```python
from build123d import *

# Parameters (mm, degrees)
SKETCH1_R           = 17.5
BOSS_EXTRUDE1_DEPTH = 10
CUT_EXTRUDE2_DEPTH  = 3
SKETCH4_R           = 17.5
CUT_EXTRUDE3_DEPTH  = 5
SKETCH5_R           = 1.6
CUT_EXTRUDE4_DEPTH  = 5


with BuildPart() as part:
    # Sketch1 → Boss-Extrude1 (new body)
    with BuildSketch(Plane(origin=(0, 0, 0), x_dir=(1, 0, 0), z_dir=(0, 1, 0))):
        with Locations(Location((0, 0, 0), (0, 0, 270))):
            Circle(SKETCH1_R)
    extrude(amount=BOSS_EXTRUDE1_DEPTH)

    # Sketch3 → Cut-Extrude2 (cut)
    with BuildSketch(Plane(origin=(-674.936170281, 10, -1288.963286539), x_dir=(1, 0, 0), z_dir=(0, 1, 0))):
        with BuildLine():
            Line((670.88481746, -1281.946137613), (662.239438243, -1279.26312032))
            add(Edge.make_bspline(
                [(662.239438243, -1279.26312032), (660.816630975, -1279.364358211), (659.786645841, -1280.216704525), (659.563484847, -1281.534870974), (660.187213896, -1282.817677158)],
                knots=[0.002399099, 0.002399099, 0.002399099, 0.375599775, 0.624400225, 0.997600901, 0.997600901, 0.997600901], degree=2))
            Line((660.187213896, -1282.817677158), (666.833464638, -1288.963286539))
            Line((666.833464638, -1288.963286539), (660.187213896, -1295.108895919))
            add(Edge.make_bspline(
                [(660.187213896, -1295.108895919), (659.563484847, -1296.391702103), (659.786645841, -1297.709868552), (660.816630975, -1298.562214867), (662.239438243, -1298.663452757)],
                knots=[0.002399099, 0.002399099, 0.002399099, 0.375599775, 0.624400225, 0.997600901, 0.997600901, 0.997600901], degree=2))
            Line((662.239438243, -1298.663452757), (670.88481746, -1295.980435464))
            Line((670.88481746, -1295.980435464), (672.883945934, -1304.809062138))
            add(Edge.make_bspline(
                [(672.883945934, -1304.809062138), (673.683024153, -1305.990630431), (674.936170281, -1306.456450565), (676.189316409, -1305.990630431), (676.988394628, -1304.809062138)],
                knots=[0.002399099, 0.002399099, 0.002399099, 0.375599775, 0.624400225, 0.997600901, 0.997600901, 0.997600901], degree=2))
            Line((676.988394628, -1304.809062138), (678.987523102, -1295.980435464))
            Line((678.987523102, -1295.980435464), (687.632902319, -1298.663452757))
            add(Edge.make_bspline(
                [(687.632902319, -1298.663452757), (689.055709587, -1298.562214867), (690.085694721, -1297.709868552), (690.308855715, -1296.391702103), (689.685126666, -1295.108895919)],
                knots=[0.002399099, 0.002399099, 0.002399099, 0.375599775, 0.624400225, 0.997600901, 0.997600901, 0.997600901], degree=2))
            Line((689.685126666, -1295.108895919), (683.038875923, -1288.963286539))
            Line((683.038875923, -1288.963286539), (689.685126666, -1282.817677158))
            add(Edge.make_bspline(
                [(689.685126666, -1282.817677158), (690.308855715, -1281.534870974), (690.08569472, -1280.216704525), (689.055709587, -1279.364358211), (687.632902319, -1279.26312032)],
                knots=[0.002399099, 0.002399099, 0.002399099, 0.375599775, 0.624400225, 0.997600901, 0.997600901, 0.997600901], degree=2))
            Line((687.632902319, -1279.26312032), (678.987523102, -1281.946137613))
            Line((678.987523102, -1281.946137613), (676.986708426, -1273.110064271))
            add(Edge.make_bspline(
                [(676.986708426, -1273.110064271), (676.173308063, -1271.410983092), (674.936170281, -1270.754606381), (673.699032499, -1271.410983092), (672.885632136, -1273.110064271)],
                knots=[0.001074269, 0.001074269, 0.001074269, 0.375268567, 0.624731433, 0.998925731, 0.998925731, 0.998925731], degree=2))
            Line((672.885632136, -1273.110064271), (670.88481746, -1281.946137613))
        make_face()
    extrude(amount=-CUT_EXTRUDE2_DEPTH, mode=Mode.SUBTRACT)

    # Sketch4 → Cut-Extrude3 (cut)
    with BuildSketch(Plane.XZ):
        with Locations(Location((0, 0, 0), (0, 0, 270))):
            Circle(SKETCH4_R)
    extrude(amount=-CUT_EXTRUDE3_DEPTH, mode=Mode.SUBTRACT)

    # Sketch5 → Cut-Extrude4 (cut)
    with BuildSketch(Plane(origin=(0, 7, 0), x_dir=(1, 0, 0), z_dir=(0, 1, 0))):
        with Locations(Location((0, 0, 0), (0, 0, 270))):
            Circle(SKETCH5_R)
    extrude(amount=-CUT_EXTRUDE4_DEPTH, mode=Mode.SUBTRACT)


solid = part.part
```
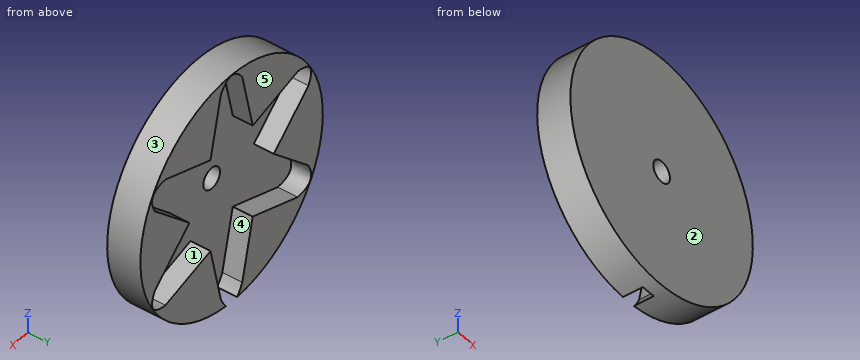
Input: part model. Units: mm. Frame: model coordinates. Face numbers are marked on the shaded views. A direction names the side the tool comes from. Coordinates: 2 decimals unless noted, no trailing zeros. Write each loop counter-clockwise with the first axis right and the second up, starting at its lowest first coordinate (ties: lowest second). Pieces come first, ordered by that corner, then holes.
1) Section D-D on z = 15. Output: boundary loops of the cut face in (x, y), and give its area (3 significant figures).
2) Section A-A on y = 5.9. Output: boundary loops of the cut face in (x, z).
3) Set-up query: the marked faces 1 and 2. Return all of +Z, -Z, +X, -X, +Y, -Y with unobstructed straight access to the full face (end or side cutting, diameter ignored); none if empty.
4) Section B-B on z = -14. Output: boundary loops of the cut face in (x, y), and give its area (3 significant figures).
5) Pin query (flat end, axial travel): pin 1 Ø1.5 at (x, z) = (11, 5.5) entering from +Y; pin 2 Ø1 at (x, y) = (6, 8) entering from +Z; pin 3 Ø3 at (y, z) = (5.5, 4.5) entering from -X. Return the tip coordinate at first contact, or that it passes through.
6) Material intervals for line 1 along X through (y, z) = (6.5, 0); line 2 along Z through (x, y) = (9, 7.55); line 3 along Z through (x, y) = (10, 9.35), sorted ascending.
7) Mould query, pull axis X, two halves, no side actions, for the marked faces 3, 4 and 5. Classes: pulls with the +X half, pulls with the -X half, needs draft (parallel to the pull), parting line crosses it, or undercut.
8) Section C-C on x = 11. Output: boundary loops of the cut face in (y, z), and give its area (3 significant figures).
Check result:
1. outline: (-9.01, 5) - (9.01, 5) - (9.01, 10) - (2.24, 10) - (2.24, 7) - (-2.24, 7) - (-2.24, 10) - (-9.01, 10) - close
1. area: 76.7 mm2
2. outline: circle Ø35 at (0, 0); hole circle Ø3.2 at (0, 0)
3. face 1: +Y
3. face 2: +Z, -Z, +X, -X, -Y
4. outline: (-10.5, 5) - (10.5, 5) - (10.5, 10) - (2.47, 10) - (2.47, 7) - (-2.47, 7) - (-2.47, 10) - (-10.5, 10) - close
4. area: 90.2 mm2
5. pin 1: stops at y = 7
5. pin 2: stops at z = 16.61
5. pin 3: stops at x = -17.24
6. line 1: x = -17.5 to -1.6, 1.6 to 17.5
6. line 2: z = -15.01 to -8.55, -0.83 to 0.83, 8.55 to 15.01
6. line 3: z = -14.36 to -8.86, -1.75 to 1.75, 8.86 to 14.36
7. face 3: parting line crosses it
7. face 4: undercut
7. face 5: needs draft
8. outline: (5, -13.61) - (10, -13.61) - (10, -9.17) - (7, -9.17) - (7, -2.68) - (10, -2.68) - (10, 2.68) - (7, 2.68) - (7, 9.17) - (10, 9.17) - (10, 13.61) - (5, 13.61) - close
8. area: 97.1 mm2
